The listing builds one solid part. Answer for the finished solid, in the listing's coordinates (mm). Face numbers are marked on the shaded views. A direction names the side the tool comes from. Give positions to 0.01 mm unless a question says otherwise; leave off trailing zeros. Write each loop counter-clockwise with the first axis right and the second up, starting at its lowest first coordinate (ties: lowest second). Pieces come first, ordered by that corner, then holes. Notation, with made-up numbers: (-39.75, 76.5) - (-30.75, 76.5) arc R27 cw to (-30.75, 102.5) - close; hole circle Ø5 at (38.25, 8.25). An arc over 180 degrees is marked (long way). One line per item, written item: value. Start each with the question number.
from build123d import *

# Parameters (mm, degrees)
F0_W     = 30
F0_H     = 30
F1_DEPTH = 5
F2_W     = 15
F2_H     = 5
F3_DEPTH = 30
F4_R     = 1
F6_D     = 5


with BuildPart() as f1:
    # F0 (on Top) → F1 (new body)
    with BuildSketch(Plane.XY):
        Rectangle(F0_W, F0_H)
    extrude(amount=-F1_DEPTH)

    # F2 (on face) → F3 (join)
    with BuildSketch(Plane(origin=(-15, 0, 0), x_dir=(0, -1, 0), z_dir=(-1, 0, 0))):
        with Locations((-22.5, 10)):
            Rectangle(F2_W, F2_H)
        with BuildLine():
            ThreePointArc((0, 0), (-8.8388347648, 3.6611652352), (-12.5, 12.5))
            Line((-12.5, 12.5), (-15, 12.5))
            Line((-15, 12.5), (-15, 7.5))
            Line((-15, 7.5), (-15, 0))
            Line((-15, 0), (0, 0))
        make_face()
        with BuildLine():
            ThreePointArc((12.5, 12.5), (8.8388347648, 3.6611652352), (0, 0))
            Line((0, 0), (15, 0))
            Line((15, 0), (15, 7.5))
            Line((15, 7.5), (15, 12.5))
            Line((15, 12.5), (12.5, 12.5))
        make_face()
        with Locations((22.5, 10)):
            Rectangle(F2_W, F2_H)
    extrude(amount=-F3_DEPTH)

    # F4
    f4_edges = [f1.edges().sort_by_distance(p)[0] for p in [
        (0, 12.5, 12.5),
        (0, -15, 7.5),
        (0, 15, 7.5),
        (0, -12.5, 12.5),
    ]]
    fillet(f4_edges, radius=F4_R)

    # F6 (through all)
    with Locations(Plane.XY.offset(12.5)):
        with Locations((0, 21.7314560089), (0, -21.7314560089)):
            Hole(F6_D / 2)


solid = f1.part
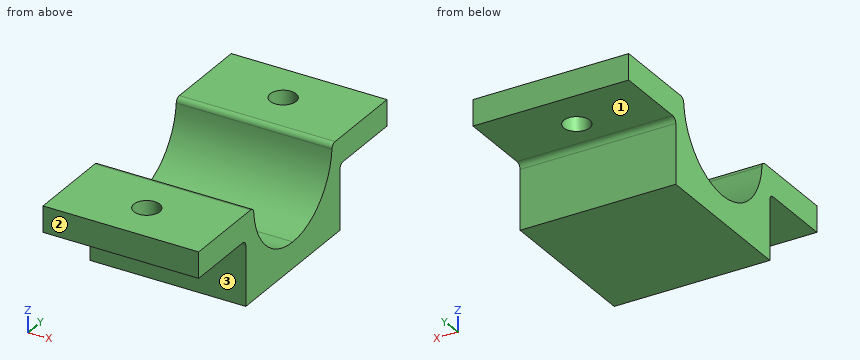
Item 1: Find section D-D on y = -18. Determine the outline of the cut face in (x, z).
Item 2: Each of these flat-tipped pins is pushed along its axis until it touches: pin 1 Ø2 at (x, y) = (4, -7.5) entering from +Z; pin 2 Ø11 at (x, y) = (6, -24) entering from -Z; pin 3 Ø3.5 at (x, z) = (-1, 2) entering from -Y; pin 4 Ø8 at (y, z) = (22.5, -0.5) entering from +X. Where does it stop, or does it pass through?
Item 3: Find section B-B on x = 0. Determine the outline of the cut face in (y, z).
Item 4: Find section A-A on z = 2.5. Determine the outline of the cut face in (x, y), plus the area to 3 significant figures.
Item 5: Straight lines are drawn through the part: line 1 along Y through (x, z) = (0, 10.6); line 2 along Y through (x, z) = (0, 11.4); line 3 along Z through (x, y) = (-5.75, -16.5). For each, find the intervals that lie inside material, in ascending order.
Item 6: For the marked faces 1, 2 and 3, determine the directions among +Z, -Z, +X, -X, +Y, -Y from which every point of the face is accessible in a straight line to the end or side of a thin tool.
Item 7: Find section C-C on x = 10. Determine the outline of the cut face in (y, z), plus the area to 3 significant figures.
Values:
1. outline: (-15, 7.5) - (15, 7.5) - (15, 12.5) - (-15, 12.5) - close
2. pin 1: z = 3.33
2. pin 2: z = 7.5
2. pin 3: y = -15
2. pin 4: through
3. outline: (-30, 7.5) - (-24.23, 7.5) - (-24.23, 12.5) - (-30, 12.5) - close; (-19.23, 7.5) - (-16, 7.5) arc R1 cw to (-15, 6.5) - (-15, -5) - (15, -5) - (15, 6.5) arc R1 cw to (16, 7.5) - (19.23, 7.5) - (19.23, 12.5) - (13.46, 12.5) arc R1 ccw to (12.47, 11.57) arc R12.5 cw to (-12.47, 11.57) arc R1 ccw to (-13.46, 12.5) - (-19.23, 12.5) - close; (24.23, 7.5) - (30, 7.5) - (30, 12.5) - (24.23, 12.5) - close
4. outline: (-15, -15) - (15, -15) - (15, -7.5) - (-15, -7.5) - close; (-15, 7.5) - (15, 7.5) - (15, 15) - (-15, 15) - close
4. area: 450 mm^2
5. line 1: -30 to -24.23, -19.23 to -12.35, 12.35 to 19.23, 24.23 to 30
5. line 2: -30 to -24.23, -19.23 to -12.45, 12.45 to 19.23, 24.23 to 30
5. line 3: 7.5 to 12.5
6. face 1: -Z, +X, -X, +Y
6. face 2: +Z, -Z, +X, -X, -Y
6. face 3: -Z, +X, -X, -Y
7. outline: (-30, 7.5) - (-16, 7.5) arc R1 cw to (-15, 6.5) - (-15, -5) - (15, -5) - (15, 6.5) arc R1 cw to (16, 7.5) - (30, 7.5) - (30, 12.5) - (13.46, 12.5) arc R1 ccw to (12.47, 11.57) arc R12.5 cw to (-12.47, 11.57) arc R1 ccw to (-13.46, 12.5) - (-30, 12.5) - close
7. area: 430 mm^2
